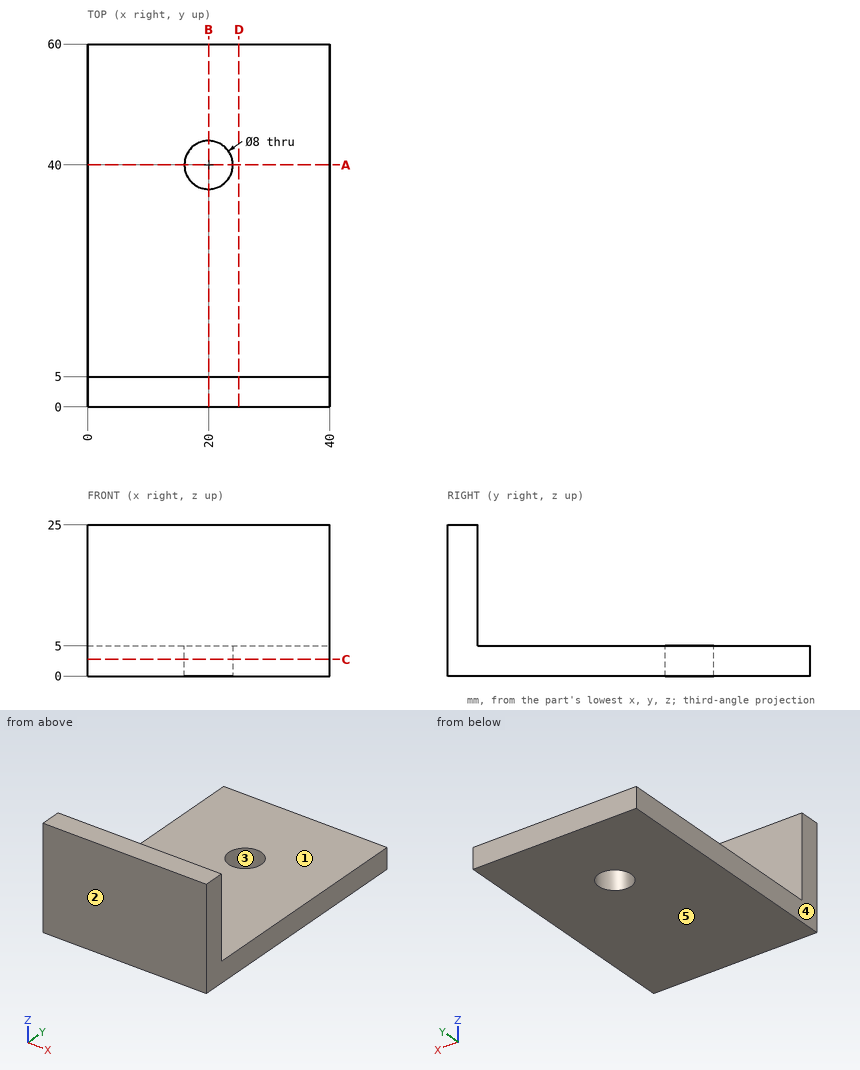
Here's the drawing with two shaded views (mm, measured from the low corner). I have some questions. A direction names the side the tool comes from. Give positions to 0.01 mm unless a question says otherwise; leave off trailing zeros. Loops run counter-clockwise (first coordinate to the right, second up) from the corner with the lowest first, then second, coordinate; pieces in that order, holes last. Notation, with made-up numbers: M 16,-14.5 L 24,-14.5 A20 ccw 24,15.5 Z; hole C -1,30.5 d5. An arc over 180 degrees is marked long. One line per item, written item: value.
1) I'm going to push a flat-ended pin straight in: pin 1 (8 mm diameter, centred on x = 11.5, z = 16.5, fed in from +Y). Where does the tip first touch, or does it pass through?
Geometry check:
pin 1: stops at y = 5
2) Please list where these lines run through material, in increasing order: line 1 (Y direction, x = 20, z = 2.05); line 2 (Z direction, x = 9.5, y = 30).
Geometry check:
line 1: y = 0 to 36, 44 to 60
line 2: z = 0 to 5
3) Imagine slicing it at B-B on x = 20. Write out the boundary of the cut face in (y, z), and give its area (3 significant figures).
Geometry check:
outline: M 0,0 L 36,0 L 36,5 L 5,5 L 5,25 L 0,25 Z; M 44,0 L 60,0 L 60,5 L 44,5 Z
area: 360 mm²
4) On a 3-axis mill with a long thin cutter (end or side, diameter ignored), from which of +Z, -Z, +X, -X, +Y, -Y can I reach the whole of each face in a straight line? I mean the marked faces 1 and 2. Say none if no direction works.
Geometry check:
face 1: +Z, +X, -X, +Y
face 2: +Z, -Z, +X, -X, -Y
5) Imagine slicing it at D-D on x = 25. Write out the boundary of the cut face in (y, z).
Geometry check:
outline: M 0,0 L 60,0 L 60,5 L 5,5 L 5,25 L 0,25 Z
6) Thinking about a two-plate mould opening in X: for the marked faces 3, 4 and 5, which applies, +X half, -X half, draft (parallel to the pull), parting line (faces both ways), or undercut?
Geometry check:
face 3: undercut
face 4: -X half
face 5: draft
7) Imagine slicing it at C-C on z = 2.75. Write out the boundary of the cut face in (x, y), and give its area (3 significant figures).
Geometry check:
outline: M 0,0 L 40,0 L 40,60 L 0,60 Z; hole C 20,40 d8
area: 2,350 mm²
8) Imagine slicing it at A-A on y = 40. Write out the boundary of the cut face in (x, z), and give its area (3 significant figures).
Geometry check:
outline: M 0,0 L 16,0 L 16,5 L 0,5 Z; M 24,0 L 40,0 L 40,5 L 24,5 Z
area: 160 mm²
